Solid Edge part; units mm, degrees
sketch "Sketch1" plane through (0, 0, 0) normal (0, 0, 1) x (1, 0, 0)
  line L0 (-72.5316, -9.9352) -> (47.4684, -9.9352)
  line L1 (47.4684, -9.9352) -> (47.4684, 50.0648)
  line L2 (47.4684, 50.0648) -> (-72.5316, 50.0648)
  line L3 (-72.5316, 50.0648) -> (-72.5316, -9.9352)
  dimension "D1" = 47.4684
  dimension "D2" = 72.5316
extrude "Protrusion1" add sketch "Sketch1" along normal blind 6
sketch "Sketch2" plane through (-52.5316, 30.0648, 6) normal (0, 0, 1) x (1, 0, 0)
  circle A0 centre (70, -10) radius 12.5
  circle A1 centre (70, -10) radius 11
extrude "ExtrudedProtrusion_2" add sketch "Sketch2" along normal blind 5
Could you check a few things on this model? Use its own coordinates, in mm. A direction names the side the tool comes from. Give positions to 0.01 mm unless a question says otherwise; leave off trailing zeros. Order: outer loops, then holes, each group sorted by start corner. A loop starts at its lowest first (then second) coordinate and runs counter-clockwise, first axis right, second up.
Item 1: If we section it at B-B, the plane y = 22.5: Write out the boundary of the cut face in (x, z), plus the area to 3 significant figures.
Item 2: For faces 4 (the face through (27.96, 16.76, 8.46)), 5 (the face through (24, 11, 11)), which set-ups out of +Z, -Z, +X, -X, +Y, -Y let a thin tool reach every point of the face, with its end or its side?
Item 3: If we mould it in two halves opening along X, with no side actions, what happens to faces 1 (the face through (17, 20, 6)), 2 (the face through (-72.532, 20, 3)), 3 (the face through (15.84, 7.67, 8.46))? For each: pulls with the +X half, pulls with the -X half, needs draft (parallel to the pull), parting line crosses it, or undercut.
Item 4: If we section it at D-D, the plane x = 40.5: Write out the boundary of the cut face in (y, z), plus the area to 3 significant figures.
Item 5: I'm going to push flat-ended pins straight in: pin 1 (11 mm diameter, centred on x = 17, y = 16.5, fed in from +Z); pin 2 (2 mm diameter, centred on x = -10, y = 20, fed in from -Z). Where does each tip first touch, or does it pass through?
Item 6: If we section it at A-A, the plane x = 21: Write out the boundary of the cut face in (y, z), plus the area to 3 significant figures.
Item 7: I need wall thicknesses on line 1 (Z direction, x = 14, y = 47.5); line 2 (Y direction, x = 9, z = 8.5); line 3 (Y direction, x = 22, z = 9). Which ranges of each line are inside material? Lowest first, please.
Item 8: If we section it at C-C, the plane y = -4.5: Write out the boundary of the cut face in (x, z).
Values:
1. outline: (-72.53, 0) - (47.47, 0) - (47.47, 6) - (29.73, 6) - (29.73, 11) - (28.2, 11) - (28.2, 6) - (6.74, 6) - (6.74, 11) - (5.21, 11) - (5.21, 6) - (-72.53, 6) - close
1. area: 735 mm2
2. face 4: +Z
2. face 5: +Z, +X, -X, +Y, -Y
3. face 1: undercut
3. face 2: pulls with the -X half
3. face 3: parting line crosses it
4. outline: (-9.94, 0) - (50.06, 0) - (50.06, 6) - (-9.94, 6) - close
4. area: 360 mm2
5. pin 1: stops at z = 6
5. pin 2: stops at z = 0
6. outline: (-9.94, 0) - (50.06, 0) - (50.06, 6) - (32.06, 6) - (32.06, 11) - (30.48, 11) - (30.48, 6) - (9.65, 6) - (9.65, 11) - (8.07, 11) - (8.07, 6) - (-9.94, 6) - close
6. area: 376 mm2
7. line 1: z = 0 to 6
7. line 2: y = 10.87 to 13.04, 27.09 to 29.26
7. line 3: y = 8.42 to 10.04, 30.09 to 31.71
8. outline: (-72.53, 0) - (47.47, 0) - (47.47, 6) - (-72.53, 6) - close
